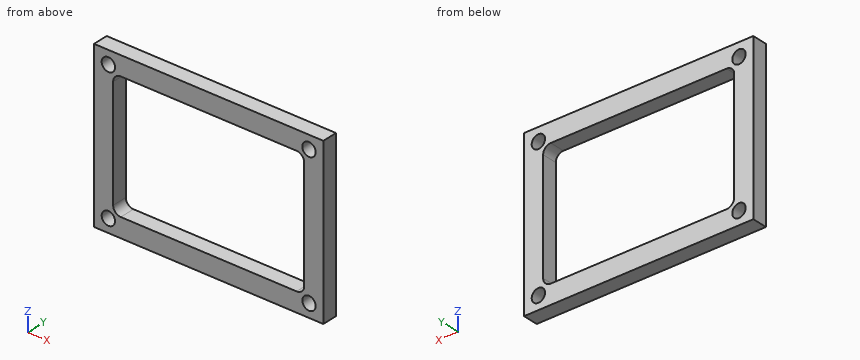
Autodesk Inventor part; units mm, degrees
ref_plane "YZ Plane" through (0, 0, 0) normal (1, 0, 0) x (0, 1, 0)
ref_plane "XZ Plane" through (0, 0, 0) normal (0, 1, 0) x (-1, 0, 0)
ref_plane "XY Plane" through (0, 0, 0) normal (0, 0, 1) x (1, 0, 0)
sketch "Boceto1" plane through (0, 0, 0) normal (0, 1, 0) x (-1, 0, 0)
  line L0 (-30, -21.5) -> (30, -21.5)
  line L1 (30, -21.5) -> (30, 21.5)
  line L2 (30, 21.5) -> (-30, 21.5)
  line L3 (-30, 21.5) -> (-30, -21.5)
  line L4 (-30, -21.5) -> (30, 21.5) construction
  line L5 (30, -21.5) -> (-30, 21.5) construction
  line L6 (-23, 16.5) -> (23, 16.5)
  line L7 (25, 14.5) -> (25, -14.5)
  line L8 (23, -16.5) -> (-23, -16.5)
  line L9 (-25, -14.5) -> (-25, 14.5)
  line L10 (30, 21.5) -> (28, 21.5)
  line L11 (28, 21.5) -> (28, -21.5)
  line L12 (-30, 21.5) -> (-28, 21.5)
  line L13 (-28, 21.5) -> (-28, -21.5)
  line L14 (30, 21.5) -> (30, 19.8)
  line L15 (30, 19.8) -> (-30, 19.8)
  line L16 (30, -21.5) -> (30, -19.8)
  line L17 (30, -19.8) -> (-30, -19.8)
  circle A0 centre (26.25, -18.05) radius 1.75
  circle A1 centre (26.25, 18.05) radius 1.75
  circle A2 centre (-26.25, 18.05) radius 1.75
  circle A3 centre (-26.25, -18.05) radius 1.75
  arc A4 (25, 14.5) -> (23, 16.5) centre (23, 14.5) ccw
  arc A5 (23, -16.5) -> (25, -14.5) centre (23, -14.5) ccw
  arc A6 (-25, -14.5) -> (-23, -16.5) centre (-23, -14.5) ccw
  arc A7 (-23, 16.5) -> (-25, 14.5) centre (-23, 14.5) ccw
  point P0 (0, 0)
  dimension "d0" = 60
  dimension "d1" = 43
  dimension "d2" = 5
  dimension "d3" = 2
  dimension "d4" = 2
  dimension "d5" = 1.7
  dimension "d6" = 1.7
  dimension "d8" = 3.5
  dimension "d9" = 3.5
  dimension "d10" = 3.5
  dimension "d11" = 3.5
  dimension "d12" = 2
  dimension "d13" = 2
extrude "Extrusión1" add sketch "Boceto1" along normal blind 4 contours L3 L17 L13 L0 | L13 L17 L11 L0 | L3 L15 L13 L17 | L11 L17 L1 L0 | L13 A3 L17 | L3 L2 L13 L15 | L17 A0 L11 | L11 L15 L1 L17 | L13 A2 L15 A1 L11 A0 L17 A3 | L15 A2 L13 | L13 L2 L11 L15 | L15 L11 L2 L1 | A1 L15 L11
properties part number "Buck 1"
CAD build for the part. Positions are in the model's coordinates, mm. Round coordinates to 2 decimals unless told otherwise and drop trailing zeros. Write each loop counter-clockwise with the first axis right and the second up, starting at its lowest first coordinate (ties: lowest second). Pieces come first, ordered by that corner, then holes. Notation, with made-up numbers: M 49,-16.5 L 72,-16.5 A37 cw 72,22.5 Z; hole C -36.75,-28 d9. An arc over 180 degrees is marked long. Put each result on its own line as item: value. Start each with the question number.
1) Saw through at D-D, the plane z = 18.05. Write the cut outline in (x, y).
2) Saw through at C-C, the plane x = -3. Write the cut outline in (y, z).
3) Saw through at B-B, the plane x = 26.25. Write the cut outline in (y, z), and give its area (3 significant figures).
4) Saw through at A-A, the plane z = 1. Write the cut outline in (x, y), and give its area (3 significant figures).
5) Drill centre lines: probe 1 along X at (y, z) = (1.65, 18.05); probe 2 along Z at (x, y) = (-26.25, 1.2); probe 3 along Z at (x, y) = (7, 1.3). Where is each one in solid material? Low to high. Write a range as [from, to].
Resolved:
1. outline: M -30,0 L -28,0 L -28,4 L -30,4 Z; M -24.5,0 L 24.5,0 L 24.5,4 L -24.5,4 Z; M 28,0 L 30,0 L 30,4 L 28,4 Z
2. outline: M 0,-21.5 L 4,-21.5 L 4,-16.5 L 0,-16.5 Z; M 0,16.5 L 4,16.5 L 4,21.5 L 0,21.5 Z
3. outline: M 0,-21.5 L 4,-21.5 L 4,-19.8 L 0,-19.8 Z; M 0,-16.3 L 4,-16.3 L 4,16.3 L 0,16.3 Z; M 0,19.8 L 4,19.8 L 4,21.5 L 0,21.5 Z
3. area: 144 mm²
4. outline: M -30,0 L -25,0 L -25,4 L -30,4 Z; M 25,0 L 30,0 L 30,4 L 25,4 Z
4. area: 40.0 mm²
5. probe 1: [-30, -28], [-24.5, 24.5], [28, 30]
5. probe 2: [-21.5, -19.8], [-16.3, 16.3], [19.8, 21.5]
5. probe 3: [-21.5, -16.5], [16.5, 21.5]
